```python
from build123d import *

# Parameters (mm, degrees)
F0_W     = 1447.8
F0_H     = 914.4
F1_DEPTH = 914.4
F2_W     = 1143
F2_H     = 685.8
F3_DEPTH = 457.2
F4_R     = 30.48


with BuildPart() as f1:
    # F0 (on Top) → F1 (new body)
    with BuildSketch(Plane.XY):
        Rectangle(F0_W, F0_H)
    extrude(amount=F1_DEPTH)

    # F2 (on face) → F3 (cut)
    with BuildSketch(Plane.XY.offset(914.4)):
        with Locations((0, -114.3)):
            Rectangle(F2_W, F2_H)
    extrude(amount=-F3_DEPTH, mode=Mode.SUBTRACT)

    # F4
    f4_edges = [f1.edges().sort_by_distance(p)[0] for p in [
        (0, -457.2, 0),
        (723.9, -457.2, 457.2),
        (647.7, -457.2, 914.4),
        (571.5, -457.2, 685.8),
        (0, -457.2, 457.2),
        (-571.5, -457.2, 685.8),
        (-647.7, -457.2, 914.4),
        (-723.9, -457.2, 457.2),
        (723.9, 457.2, 457.2),
        (723.9, 0, 0),
        (723.9, 0, 914.4),
        (-723.9, 0, 914.4),
        (0, 457.2, 914.4),
        (571.5, -114.3, 914.4),
        (0, 228.6, 914.4),
        (-571.5, -114.3, 914.4),
        (571.5, -114.3, 457.2),
        (0, 228.6, 457.2),
        (-571.5, -114.3, 457.2),
        (571.5, 228.6, 685.8),
        (-571.5, 228.6, 685.8),
        (-723.9, 457.2, 457.2),
        (-723.9, 0, 0),
        (0, 457.2, 0),
    ]]
    fillet(f4_edges, radius=F4_R)


solid = f1.part
```
Build history of the part. All positions in model axes, mm. A direction names the side the tool comes from. Round coordinates to 2 decimals unless told otherwise and drop trailing zeros. Write each loop counter-clockwise with the first axis right and the second up, starting at its lowest first coordinate (ties: lowest second). Pieces come first, ordered by that corner, then holes.
1) Drill centre lines: probe 1 along X at (y, z) = (-259, 805); probe 2 along Y at (x, z) = (84, 536); probe 3 along Z at (x, y) = (-367, 153). Where is each one in solid material? Low to high.
2) 3-axis set-ups, long thin cutter, end or side, ignore diameter. For faces 1 (the flat face through (-8, 228.6, 689)), 2 (the cylindrical face through (714.73, 5.97, 905.71)): which of +Z, -Z, +X, -X, +Y, -Y reach the whole face in a straight line?
3) Band-saw the part on A-A, the plane y = -173.5. List the corners of the cut face in (x, z).
4) Mould opens along X. For faces 3 (the flat face through (-10, 290, 914.4)), 4 (the cylindrical face through (714.73, 5.97, 8.69)), 5 (the cylindrical face through (7.57, 219.43, 465.89)) say: +X half, -X half, draft (parallel to the pull), parting line (faces both ways), or undercut.
5) Band-saw the part on C-C, the plane z = 628. List the corners of the cut face in (x, y).
6) Pin check, flat tip, straight feed: pin 1 (8 mm diameter, centred on x = 216, y = -341, fed in from +Z). Stop position of the tip, or through.
7) Band-saw the part on B-B, the plane x = 226. List the corners of the cut face in (y, z).
Ans:
1. probe 1: x = -723.9 to -571.5, 571.5 to 723.9
1. probe 2: y = 228.6 to 457.2
1. probe 3: z = 0 to 457.2
2. face 1: +Z, -Y
2. face 2: +Z, +X, +Y, -Y
3. outline: (-723.9, 30.48) arc R30.48 ccw to (-693.42, 0) - (693.42, 0) arc R30.48 ccw to (723.9, 30.48) - (723.9, 883.92) arc R30.48 ccw to (693.42, 914.4) - (601.98, 914.4) arc R30.48 ccw to (571.5, 883.92) - (571.5, 487.68) arc R30.48 cw to (541.02, 457.2) - (-541.02, 457.2) arc R30.48 cw to (-571.5, 487.68) - (-571.5, 883.92) arc R30.48 ccw to (-601.98, 914.4) - (-693.42, 914.4) arc R30.48 ccw to (-723.9, 883.92) - close
4. face 3: draft
4. face 4: +X half
4. face 5: undercut
5. outline: (-723.9, -426.72) arc R30.48 ccw to (-693.42, -457.2) - (-601.98, -457.2) arc R30.48 ccw to (-571.5, -426.72) - (-571.5, 198.12) arc R30.48 cw to (-541.02, 228.6) - (541.02, 228.6) arc R30.48 cw to (571.5, 198.12) - (571.5, -426.72) arc R30.48 ccw to (601.98, -457.2) - (693.42, -457.2) arc R30.48 ccw to (723.9, -426.72) - (723.9, 426.72) arc R30.48 ccw to (693.42, 457.2) - (-693.42, 457.2) arc R30.48 ccw to (-723.9, 426.72) - close
6. pin 1: stops at z = 457.2
7. outline: (-457.2, 30.48) arc R30.48 ccw to (-426.72, 0) - (426.72, 0) arc R30.48 ccw to (457.2, 30.48) - (457.2, 883.92) arc R30.48 ccw to (426.72, 914.4) - (259.08, 914.4) arc R30.48 ccw to (228.6, 883.92) - (228.6, 487.68) arc R30.48 cw to (198.12, 457.2) - (-426.72, 457.2) arc R30.48 ccw to (-457.2, 426.72) - close
